Design review of the part shown in the three views and the two pictorial views. Dimensions are in mm from the part's minimum x, y and z. A direction names the side the tool comes from. Round coordinates to 2 decimals unless told otherwise and drop trailing zeros. Loops run counter-clockwise (first coordinate to the right, second up) from the corner with the lowest first, then second, coordinate; pieces in that order, holes last. Notation, with made-up numbers: M 2,39.25 L 11,39.25 A24 cw 11,67.25 Z; hole C 7.5,-33 d2. An arc over 180 degrees is marked long. Return JSON: item names as keys, results as strings. Group by question number.
Q1. Clearance check with flat-ended pins moving along their axes: pin 1 Ø10 at (x, y) = (205, 116.5) entering from -Z; pin 2 Ø1 at (x, z) = (282, 493) entering from -Y; pin 3 Ø4 at (x, z) = (286, 167) entering from -Y. State where each tip first meets the part, or that it passes through.
Q2. For the marked faces 1, 2, 3 and 4, list the 3-axis set-ups (+Z, -Z, +X, -X, +Y, -Y) from which the entire face can be reached by the end or side of a thin tool; tool diameter is ignored.
Q3. Consider section C-C (z = 665.5). State the section outline as (x, y) points, and give its area (3 significant figures).
Q4. Consider section B-B (y = 144.5). State the section outline as (x, z) points.
Q5. To check wall thickness, follow line 1 along Y through (x, z) = (88, 145.5); line 2 along Z through (x, y) = (133, 127). State the ranges of each line that lie inside material, in increasing order.
Q6. Consider section A-A (x = 158.5). State the section outline as (y, z) points.
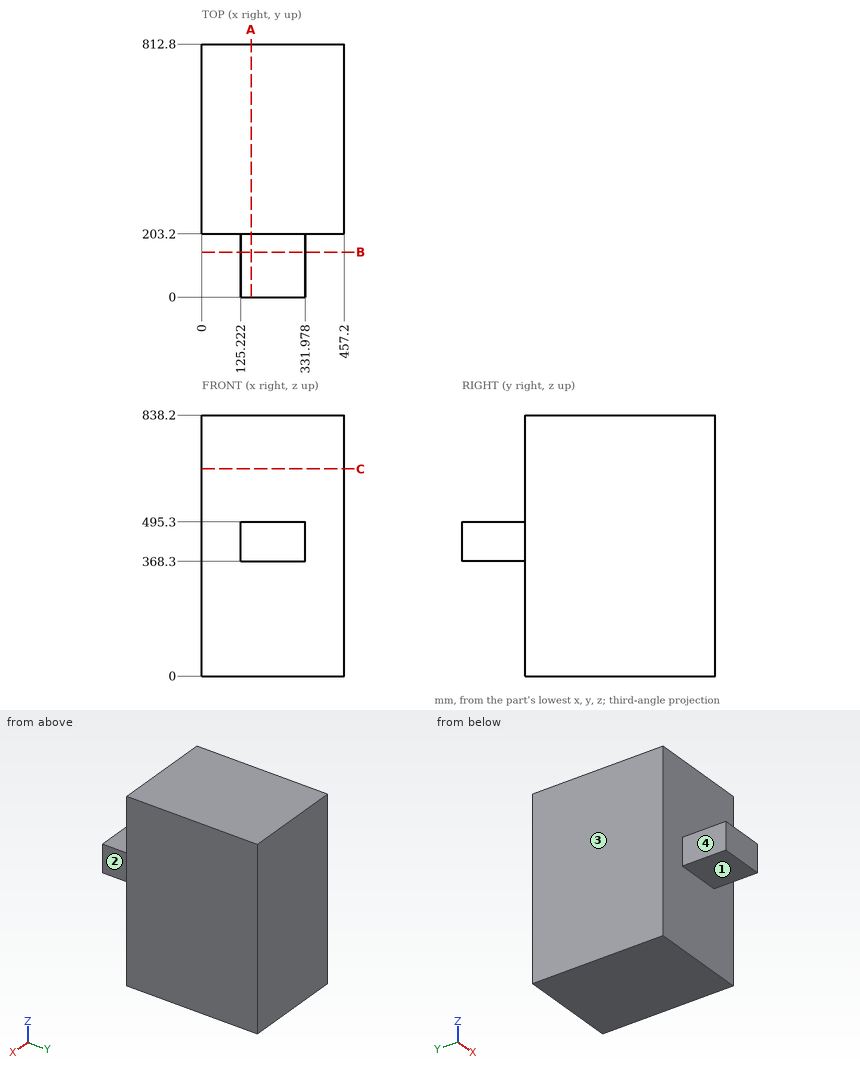
Values:
{
 "1": {"pin 1": "stops at z = 368.3", "pin 2": "stops at y = 0", "pin 3": "stops at y = 203.2"},
 "2": {"face 1": "-Z, +X, -X, -Y", "face 2": "+Z, -Z, +X, -Y", "face 3": "+Z, -Z, -X, +Y, -Y", "face 4": "+Z, -Z, -X, -Y"},
 "3": {"outline": "M 0,203.2 L 457.2,203.2 L 457.2,812.8 L 0,812.8 Z", "area": "279,000 mm2"},
 "4": {"outline": "M 125.22,368.3 L 331.98,368.3 L 331.98,495.3 L 125.22,495.3 Z"},
 "5": {"line 1": "y = 203.2 to 812.8", "line 2": "z = 368.3 to 495.3"},
 "6": {"outline": "M 0,368.3 L 203.2,368.3 L 203.2,0 L 812.8,0 L 812.8,838.2 L 203.2,838.2 L 203.2,495.3 L 0,495.3 Z"}
}
